Work out the finished part from the listing and answer in its coordinate system (mm). Face numbers are marked on the shaded views. A direction names the side the tool comes from. Coordinates: 2 decimals unless noted, no trailing zeros. Write each loop counter-clockwise with the first axis right and the second up, starting at its lowest first coordinate (ties: lowest second). Pieces come first, ordered by that corner, then holes. Notation, with made-up numbers: (-23, -2) - (20, -2) arc R11 cw to (20, 7) - close; hole circle Ø11 at (-20.75, -5). An arc over 180 degrees is marked (long way). Answer as a JSON object with one key per item and string values. Group by question number.
from build123d import *

# Parameters (mm, degrees)
SKETCH1_W            = 46
SKETCH1_H            = 33
BOSS_EXTRUDE1_DEPTH  = 23
CUT_EXTRUDE2_DEPTH   = 20
BOSS_EXTRUDE2_DEPTH  = 3
MIRROR2_COPY_1_DEPTH = 3
SKETCH6_W            = 6
SKETCH6_H            = 21
CUT_EXTRUDE3_DEPTH   = 20
SKETCH7_R            = 3
CUT_EXTRUDE5_DEPTH   = 37.47259245
SKETCH8_W            = 46
SKETCH8_H            = 3
BOSS_EXTRUDE3_DEPTH  = 6.5
SKETCH10_W           = 6
SKETCH10_H           = 21
BOSS_EXTRUDE4_DEPTH  = 20
CUT_EXTRUDE7_REACH   = 58.338
SKETCH11_W           = 21
SKETCH11_H           = 20
SKETCH13_W           = 46
SKETCH13_H           = 3
BOSS_EXTRUDE6_DEPTH  = 6.5
CUT_EXTRUDE8_DEPTH   = 1.5
SKETCH14_W           = 59
SKETCH14_H           = 3
BOSS_EXTRUDE7_DEPTH  = 6
SKETCH15_W           = 13
SKETCH15_H           = 0.75
CUT_EXTRUDE9_DEPTH   = 1.5
BOSS_EXTRUDE8_DEPTH  = 23
CUT_EXTRUDE11_REACH  = 71.016
SKETCH17_R           = 9.5
SKETCH17_W           = 57
SKETCH17_H           = 13.5
SKETCH20_W           = 53
SKETCH20_H           = 3.5
BOSS_EXTRUDE10_DEPTH = 11
SKETCH22_W           = 53
SKETCH22_H           = 1.5
CUT_EXTRUDE12_DEPTH  = 4
SKETCH23_W           = 12
SKETCH23_H           = 33
CUT_EXTRUDE13_DEPTH  = 20
SKETCH25_W           = 6.5
SKETCH25_H           = 21
BOSS_EXTRUDE11_DEPTH = 2
SKETCH27_W           = 53
SKETCH27_H           = 1
BOSS_EXTRUDE12_DEPTH = 12
SKETCH18_W           = 53
SKETCH18_H           = 1
BOSS_EXTRUDE13_DEPTH = 23
SKETCH33_W           = 12.5
SKETCH33_H           = 21
BOSS_EXTRUDE14_DEPTH = 2
CUT_EXTRUDE14_REACH  = 71.649
SKETCH34_W           = 4.5
SKETCH34_H           = 10


with BuildPart() as part:
    # Sketch1 → Boss-Extrude1 (new body)
    with BuildSketch(Plane(origin=(0, 0, 0), x_dir=(1, 0, 0), z_dir=(0, 1, 0))):
        Rectangle(SKETCH1_W, SKETCH1_H)
    extrude(amount=BOSS_EXTRUDE1_DEPTH)

    # Sketch3 → Cut-Extrude2 (cut)
    with BuildSketch(Plane.XZ):
        Polygon((-17, -10.5), (-17, -16.5), (5, -16.5), (5, -10.5), (17, -10.5), (17, 10.5), (5, 10.5), (5, 16.5), (-17, 16.5), (-17, 10.5), (-23, 10.5), (-23, -10.5), align=None)
    extrude(amount=-CUT_EXTRUDE2_DEPTH, mode=Mode.SUBTRACT)

    # Sketch5 → Boss-Extrude2 (add)
    with BuildSketch(Plane.XZ):
        Polygon((-17, 13.5), (-20, 13.5), (-20, 10.5), (-23, 10.5), (-23, 16.5), (-17, 16.5), align=None)
    boss_extrude2 = extrude(amount=BOSS_EXTRUDE2_DEPTH)

    # Mirror1: Boss-Extrude2 across plane
    add(boss_extrude2.mirror(Plane.XY))

    # Mirror2: Boss-Extrude2 across plane
    add(boss_extrude2.mirror(Plane(origin=(0, 0, 0), x_dir=(0, 0, 1), z_dir=(1, 0, 0))))

    # Mirror2 copy 1 sketch → Mirror2 copy 1 (add)
    with BuildSketch(Plane(origin=(0, 0, 0), x_dir=(-1, 0, 0), z_dir=(0, -1, 0))):
        Polygon((-17, 13.5), (-20, 13.5), (-20, 10.5), (-23, 10.5), (-23, 16.5), (-17, 16.5), align=None)
    extrude(amount=MIRROR2_COPY_1_DEPTH)

    # Sketch6 → Cut-Extrude3 (cut)
    with BuildSketch(Plane.XZ):
        with Locations((20, 0)):
            Rectangle(SKETCH6_W, SKETCH6_H)
    extrude(amount=-CUT_EXTRUDE3_DEPTH, mode=Mode.SUBTRACT)

    # Sketch7 → Cut-Extrude5 (cut, through all)
    with BuildSketch(Plane.XZ.offset(-20)):
        with Locations(Location((0, 0, 0), (0, 0, 270))):
            Circle(SKETCH7_R)
    extrude(amount=-CUT_EXTRUDE5_DEPTH, mode=Mode.SUBTRACT)

    # Sketch8 → Boss-Extrude3 (add)
    with BuildSketch(Plane(origin=(0, 0, -16.5), x_dir=(-1, 0, 0), z_dir=(0, 0, -1))):
        with Locations((0, 21.5)):
            Rectangle(SKETCH8_W, SKETCH8_H)
    boss_extrude3 = extrude(amount=BOSS_EXTRUDE3_DEPTH)

    # Mirror3: Boss-Extrude3 across plane
    add(boss_extrude3.mirror(Plane.XY))

    # Sketch10 → Boss-Extrude4 (add)
    with BuildSketch(Plane.XZ.offset(-20)):
        with Locations((-20, 0)):
            Rectangle(SKETCH10_W, SKETCH10_H)
    extrude(amount=BOSS_EXTRUDE4_DEPTH)

    # Sketch11 → Cut-Extrude7 (cut, up to next)
    with BuildSketch(Plane.ZY.offset(23), mode=Mode.PRIVATE) as cut_extrude7_sk1:
        with Locations((0, 8)):
            Rectangle(SKETCH11_W, SKETCH11_H)
    cut_extrude7_tool1 = extrude(cut_extrude7_sk1.sketch, amount=-CUT_EXTRUDE7_REACH, mode=Mode.PRIVATE) & part.part
    add(cut_extrude7_tool1.solids().sort_by_distance((-23, 8, 0))[0], mode=Mode.SUBTRACT)

    # Sketch13 → Boss-Extrude6 (add)
    with BuildSketch(Plane(origin=(23, 0, 0), x_dir=(0, 0, -1), z_dir=(1, 0, 0))):
        with Locations((0, 21.5)):
            Rectangle(SKETCH13_W, SKETCH13_H)
    boss_extrude6 = extrude(amount=BOSS_EXTRUDE6_DEPTH)

    # Mirror4: Boss-Extrude6 across plane
    add(boss_extrude6.mirror(Plane(origin=(0, 0, 0), x_dir=(0, 0, 1), z_dir=(1, 0, 0))))

    # Sketch12 → Cut-Extrude8 (cut)
    with BuildSketch(Plane.XZ.offset(-20)):
        Polygon((-6.5, -20.5), (-6.5, -23), (6.5, -23), (6.5, -20.5), (26, -20.5), (26, -19), (-26, -19), (-26, -20.5), align=None)
    extrude(amount=-CUT_EXTRUDE8_DEPTH, mode=Mode.SUBTRACT)

    # Sketch14 → Boss-Extrude7 (add)
    with BuildSketch(Plane(origin=(0, 0, -23), x_dir=(-1, 0, 0), z_dir=(0, 0, -1))):
        with Locations((0, 21.5)):
            Rectangle(SKETCH14_W, SKETCH14_H)
    boss_extrude7 = extrude(amount=BOSS_EXTRUDE7_DEPTH)

    # Mirror5: Boss-Extrude7 across plane
    add(boss_extrude7.mirror(Plane.XY))

    # Sketch15 → Cut-Extrude9 (cut)
    with BuildSketch(Plane.XZ.offset(-20)):
        with Locations((0, -23.375)):
            Rectangle(SKETCH15_W, SKETCH15_H)
    extrude(amount=-CUT_EXTRUDE9_DEPTH, mode=Mode.SUBTRACT)

    # Sketch16 → Boss-Extrude8 (add)
    with BuildSketch(Plane.XZ.offset(-20)):
        Polygon((-28.5, 28), (-26.5, 28), (-26.5, 29), (-29.5, 29), (-29.5, 10.5), (-28.5, 10.5), align=None)
        Polygon((26.5, 28), (28.5, 28), (28.5, 10.5), (29.5, 10.5), (29.5, 29), (26.5, 29), align=None)
        Polygon((29.5, -10.5), (28.5, -10.5), (28.5, -28), (-28.5, -28), (-28.5, -10.5), (-29.5, -10.5), (-29.5, -29), (29.5, -29), align=None)
    extrude(amount=BOSS_EXTRUDE8_DEPTH)

    # Sketch17 → Cut-Extrude11 (cut, up to next)
    with BuildSketch(Plane(origin=(0, 0, -29), x_dir=(-1, 0, 0), z_dir=(0, 0, -1)), mode=Mode.PRIVATE) as cut_extrude11_sk1:
        with Locations((13, 10.5)):
            Circle(SKETCH17_R)
    cut_extrude11_tool1 = extrude(cut_extrude11_sk1.sketch, amount=-CUT_EXTRUDE11_REACH, mode=Mode.PRIVATE) & part.part
    # Sketch17 → Cut-Extrude11 (cut, up to next)
    with BuildSketch(Plane(origin=(0, 0, -29), x_dir=(-1, 0, 0), z_dir=(0, 0, -1)), mode=Mode.PRIVATE) as cut_extrude11_sk2:
        with Locations((-13, 10.5)):
            Circle(SKETCH17_R)
    cut_extrude11_tool2 = extrude(cut_extrude11_sk2.sketch, amount=-CUT_EXTRUDE11_REACH, mode=Mode.PRIVATE) & part.part
    # Sketch17 → Cut-Extrude11 (cut, up to next)
    with BuildSketch(Plane(origin=(0, 0, -29), x_dir=(-1, 0, 0), z_dir=(0, 0, -1)), mode=Mode.PRIVATE) as cut_extrude11_sk3:
        with Locations((0, 3.75)):
            Rectangle(SKETCH17_W, SKETCH17_H)
    cut_extrude11_tool3 = extrude(cut_extrude11_sk3.sketch, amount=-CUT_EXTRUDE11_REACH, mode=Mode.PRIVATE) & part.part
    add(cut_extrude11_tool1.solids().sort_by_distance((-13, 10.5, -29))[0], mode=Mode.SUBTRACT)
    add(cut_extrude11_tool2.solids().sort_by_distance((13, 10.5, -29))[0], mode=Mode.SUBTRACT)
    add(cut_extrude11_tool3.solids().sort_by_distance((0, 3.75, -29))[0], mode=Mode.SUBTRACT)

    # Sketch20 → Boss-Extrude10 (add)
    with BuildSketch(Plane.XZ.offset(-20)):
        with Locations((0, 20.25)):
            Rectangle(SKETCH20_W, SKETCH20_H)
    extrude(amount=BOSS_EXTRUDE10_DEPTH)

    # Sketch22 → Cut-Extrude12 (cut)
    with BuildSketch(Plane.XZ.offset(-9)):
        with Locations((0, 20.25)):
            Rectangle(SKETCH22_W, SKETCH22_H)
    extrude(amount=-CUT_EXTRUDE12_DEPTH, mode=Mode.SUBTRACT)

    # Sketch23 → Cut-Extrude13 (cut)
    with BuildSketch(Plane.XZ):
        with Locations((11, 0)):
            Rectangle(SKETCH23_W, SKETCH23_H)
    extrude(amount=-CUT_EXTRUDE13_DEPTH, mode=Mode.SUBTRACT)

    # Sketch25 → Boss-Extrude11 (add)
    with BuildSketch(Plane.XZ.offset(-20)):
        with Locations((-26.25, 0)):
            Rectangle(SKETCH25_W, SKETCH25_H)
    extrude(amount=BOSS_EXTRUDE11_DEPTH)

    # Sketch27 → Boss-Extrude12 (add)
    with BuildSketch(Plane.XZ.offset(-9)):
        with Locations((0, 21.5)):
            Rectangle(SKETCH27_W, SKETCH27_H)
    extrude(amount=BOSS_EXTRUDE12_DEPTH)

    # Sketch18 → Boss-Extrude13 (add)
    with BuildSketch(Plane.XZ.offset(-20)):
        with Locations((0, 28.5)):
            Rectangle(SKETCH18_W, SKETCH18_H)
    extrude(amount=BOSS_EXTRUDE13_DEPTH)

    # Sketch33 → Boss-Extrude14 (add)
    with BuildSketch(Plane.XZ.offset(-20)):
        with Locations((23.25, 0)):
            Rectangle(SKETCH33_W, SKETCH33_H)
    extrude(amount=BOSS_EXTRUDE14_DEPTH)

    # Sketch34 → Cut-Extrude14 (cut, up to next)
    with BuildSketch(Plane.ZY.offset(29.5), mode=Mode.PRIVATE) as cut_extrude14_sk1:
        with Locations((18.75, 2)):
            Rectangle(SKETCH34_W, SKETCH34_H)
    cut_extrude14_tool1 = extrude(cut_extrude14_sk1.sketch, amount=-CUT_EXTRUDE14_REACH, mode=Mode.PRIVATE) & part.part
    add(cut_extrude14_tool1.solids().sort_by_distance((-29.5, 2, 18.75))[0], mode=Mode.SUBTRACT)


solid = part.part
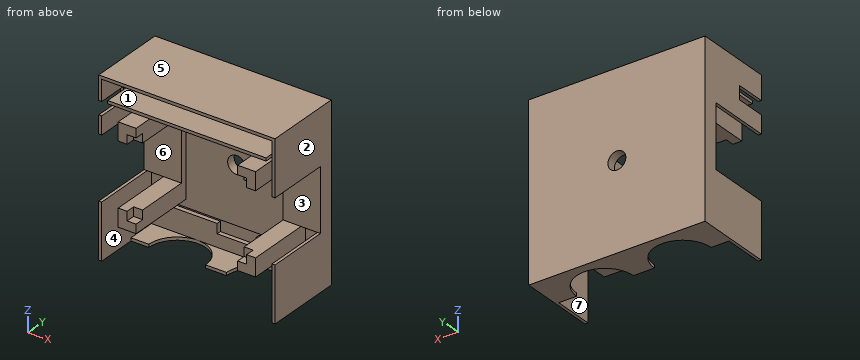
Q1. Flat-ended cylindrical pins translate along their axes: pin 1 Ø1 at (x, y) = (-9.5, 3.5) entering from -Z; pin 2 Ø0.9 at (x, z) = (18, 11.5) entering from -Y; pin 3 Ø2 at (x, y) = (12, 16) entering from -Z. Find the tip coordinate at first contact, or state that the pin passes through.
Q2. Section A-A on z = 0 is taken. Determine the outline of the cut face in (x, y), plus the area to 3 significant figures.
Q3. Section B-B on x = 0 is taken. Determine the outline of the cut face in (y, z), plus the area to 3 significant figures.
Q4. For a pull along X with two mould halves and no side action, classify the marked faces 1, 2, 3 and 4 as +X half, -X half, draft (parallel to the pull), parting line (faces both ways), or undercut.
Q5. Section C-C on y = 8 is taken. Count the separate pieces of the cut face and the enclosed holes in it, plus the area to 3 significant figures.
Q6. Consider L1, parallel to Z at x = 2, y = 15.25; L2, parallel to Z at x = -18, y = 14.75; L3, parallel to Z at x = 6, y = 10.5. Determine where each line is inside the solid, lowest interval first. Write a range as from..to.
Q7. A tool of negligible diameter and unlimited length cuts with its end or side. For the marked faces 5, 6 and 7, from which of +Z, -Z, +X, -X, +Y, -Y can it reach the whole face along a straight path? Write none if from no direction.
Q8. Section D-D on z = -22 is taken. Determine the outline of the cut face in (x, y).
Numbers:
{
 "1": {"pin 1": "stops at z = 21", "pin 2": "stops at y = 0", "pin 3": "stops at z = 18.5"},
 "2": {"outline": "(-29.5, 18) - (-17, 18) - (-17, 20) - (-3, 20) - (-3, 23) - (-29.5, 23) - close; (3, 20) - (17, 20) - (17, 18) - (29.5, 18) - (29.5, 23) - (3, 23) - close", "area": "209 mm²"},
 "3": {"outline": "(-3, 21) - (13, 21) - (13, 19.5) - (9, 19.5) - (9, 18.5) - (20, 18.5) - (20, 3) - (23, 3) - (23, 29) - (-3, 29) - (-3, 28) - (20, 28) - (20, 22) - (-3, 22) - close; (10.5, -29) - (23, -29) - (23, -3) - (20, -3) - (20, -19) - (21.5, -19) - (21.5, -23.75) - (20, -23.75) - (20, -28) - (10.5, -28) - close", "area": "226 mm²"},
 "4": {"face 1": "undercut", "face 2": "+X half", "face 3": "draft", "face 4": "undercut"},
 "5": {"separate pieces": "8", "enclosed holes": "0", "area": "328 mm²"},
 "6": {"L1": "z = -29..-28, 18.5..22, 28..29", "L2": "z = -16.5..-10.5, 10.5..16.5, 18.5..22, 28..29", "L3": "z = 18.5..19.5, 21..22, 28..29"},
 "7": {"face 5": "+Z, +X, -X, +Y, -Y", "face 6": "+X, -X, -Y", "face 7": "-Y"},
 "8": {"outline": "(-29.5, -3) - (-28.5, -3) - (-28.5, 20) - (-6.5, 20) - (-6.5, 21.5) - (6.5, 21.5) - (6.5, 20) - (28.5, 20) - (28.5, -3) - (29.5, -3) - (29.5, 23) - (-29.5, 23) - close"}
}
